Input: part model. Units: mm. Frame: model coordinates. A direction names the side the tool comes from. Round coordinates to 2 decimals unless told otherwise and drop trailing zeros. Order: outer loops, then holes, each group sorted by start corner. A loop starts at its lowest first (then second) coordinate and runs counter-clockwise, first axis right, second up.
Item 1: Cut plane B-B on x = -3.75. Output: boundary loops of the cut face in (y, z) (3 decimals), then the cut area to 3 significant figures.
Item 2: Reachability of faces 1 (the flat face through (0, -9.375, 2)), 2 (the flat face through (-4.875, 4, 13)), 3 (the flat face through (-0.375, 6, 17)) from +Z, -Z, +X, -X, +Y, -Y: full face, straight path, thin tool, end or side. Return the list, or none.
Item 3: First-contact query: pin 1 (3.5 mm diameter, centred on x = -8, y = 2, fed in from +Z); pin 2 (4.5 mm diameter, centred on y = 2.5, z = 15.5, fed in from -X) (3 decimals); pin 3 (2.5 mm diameter, centred on y = 4.5, z = 17.5, fed in from +X) (3 decimals); pin 4 (8 mm diameter, centred on x = -5, y = 2.5, fed in from -Z). Flat tips, straight axial feed; report the tip coordinate or a pass-through.
Item 4: Cut plane C-C on y = -1.25. Output: boundary loops of the cut face in (x, z) (3 decimals), then the cut area to 3 significant figures.
Item 5: Cut plane A-A on y = 7. Output: boundary loops of the cut face in (x, z) (3 decimals).
Item 6: Line query: L1, parallel to X at y = -7.5, z = 5 (3 decimals); L2, parallel to X at y = 1.25, z = 12 (3 decimals); L3, parallel to Y at x = -1, z = 12 (3 decimals). Output: solid intervals per line, ascending.
Item 7: Cut plane D-D on z = 7. Output: boundary loops of the cut face in (x, y) (3 decimals), then the cut area to 3 significant figures.
Autodesk Inventor part; units mm, degrees
ref_plane "YZ Plane" through (0, 0, 0) normal (1, 0, 0) x (0, 1, 0)
ref_plane "XZ Plane" through (0, 0, 0) normal (0, 1, 0) x (-1, 0, 0)
ref_plane "XY Plane" through (0, 0, 0) normal (0, 0, 1) x (1, 0, 0)
sketch "Sketch1" plane through (0, 0, 0) normal (0, 0, 1) x (1, 0, 0)
  line L0 (-9.375, -9.375) -> (9.375, -9.375)
  line L1 (9.375, -9.375) -> (9.375, 9.375)
  line L2 (9.375, 9.375) -> (-9.375, 9.375)
  line L3 (-9.375, 9.375) -> (-9.375, -9.375)
  line L4 (-9.375, -9.375) -> (9.375, 9.375) construction
  line L5 (9.375, -9.375) -> (-9.375, 9.375) construction
  point P0 (0, 0)
  dimension "d0" = 18.75
  dimension "d1" = 18.75
extrude "Extrusion1" add sketch "Sketch1" along normal blind 18.75
sketch "Sketch2" plane through (9.375, -9.375, 0) normal (1, 0, 0) x (0, 0, -1)
  line L0 (0, 0) -> (-4.75, 0)
  line L1 (0, 0) -> (-18.75, 0)
  line L2 (-18.75, 18.6787) -> (-18.75, 14.1787)
  line L3 (-18.75, 0) -> (-18.75, 18.75)
  line L4 (-18.75, 14.1787) -> (-4.75, 0)
  line L5 (0, 0) -> (0, 18.6787)
  line L6 (0, 18.6787) -> (-18.75, 18.6787)
  line L7 (-18.75, 0) -> (-4.75, 0)
  line L8 (-18.75, 0) -> (-18.75, 14.1787)
  point P0 (0, 9.375)
  point P1 (-18.75, 18.75)
  dimension "d4" = 4.75
  dimension "d5" = 4.5
  dimension "d6" = 45.363
  dimension "d7" = 90.001
extrude "Extrusion2" cut sketch "Sketch2" against normal blind 21 contours L1 L3 L4
sketch "Sketch3" plane through (-9.375, -9.375, 0) normal (0, -1, 0) x (1, 0, 0)
  line L0 (18.75, 18.75) -> (0, 18.75)
  line L1 (0, 18.75) -> (4.5, 18.75)
  line L2 (4.5, 18.75) -> (4.5, 9.5)
  line L3 (4.5, 9.5) -> (0, 9.5)
  line L4 (0, 9.5) -> (0, 18.75)
  line L5 (4.5, 18.75) -> (9, 18.75) construction
  line L6 (9, 18.75) -> (9, 14.25)
  line L7 (0, 0) -> (18.75, 0) construction
  line L8 (18.75, 0) -> (18.75, 4.75) construction
  line L9 (18.75, 0) -> (18.75, 18.75) construction
  line L10 (18.75, 4.75) -> (9, 14.25)
  line L11 (9, 18.75) -> (18.75, 18.75)
  line L12 (18.75, 4.75) -> (18.75, 18.75)
  point P0 (9.375, 0)
  dimension "d10" = 4.5
  dimension "d11" = 9.25
  dimension "d12" = 4.5
  dimension "d13" = 4.5
  dimension "d14" = 4.75
extrude "Extrusion3" cut sketch "Sketch3" against normal blind 27.25
From the geometry:
1. outline: (-9.375, 0) - (9.375, 0) - (9.375, 18.75) - (4.804, 18.75) - (-9.375, 4.75) - close
1. area: 252 mm2
2. face 1: +Z, -Z, +X, -X, -Y
2. face 2: +Z, -X, +Y, -Y
2. face 3: +Z, +X, +Y, -Y
3. pin 1: stops at z = 9.5
3. pin 2: stops at x = -4.875
3. pin 3: stops at x = -0.375
3. pin 4: stops at z = 0
4. outline: (-9.375, 0) - (9.375, 0) - (9.375, 4.75) - (1.141, 12.773) - (-4.875, 12.773) - (-4.875, 9.5) - (-9.375, 9.5) - close
4. area: 192 mm2
5. outline: (-9.375, 0) - (9.375, 0) - (9.375, 4.75) - (-0.375, 14.25) - (-0.375, 18.75) - (-4.875, 18.75) - (-4.875, 9.5) - (-9.375, 9.5) - close
6. L1: x = -9.375 to 9.118
6. L2: x = -4.875 to 1.934
6. L3: y = -2.032 to 9.375
7. outline: (-9.375, -7.096) - (7.066, -7.096) - (7.066, 9.375) - (-9.375, 9.375) - close
7. area: 271 mm2
